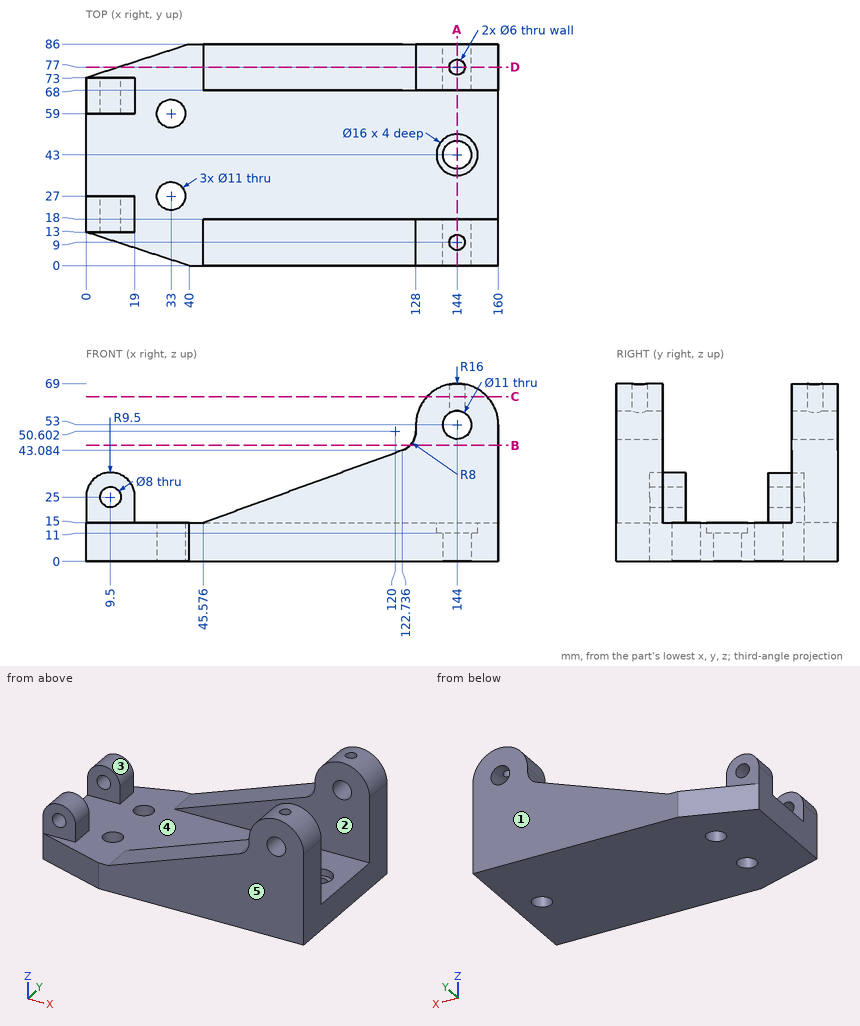
Part print with two shaded views. Sizes in mm from the minimum x, y, z corner. A direction names the side the tool comes from. Coordinates: 2 decimals unless noted, no trailing zeros. Loops run counter-clockwise (first coordinate to the right, second up) from the corner with the lowest first, then second, coordinate; pieces in that order, holes last. Notation, with made-up numbers: (-31.75, 77) -> (-22.75, 77) arc R13 cw to (-22.75, 81) -> close; hole circle Ø3 at (84.5, 21.25). An arc over 180 degrees is marked (long way). Answer as a JSON object with one key per item and string values.
Q1. Cut at B-B (z = 45). List the corners of the cut face in (x, y), and give its area (3 significant figures).
Report:
{"outline": "(125.71, 0) -> (160, 0) -> (160, 18) -> (125.71, 18) -> close; (125.71, 68) -> (160, 68) -> (160, 86) -> (125.71, 86) -> close", "area": "1,230 mm2"}
Q2. Cut at D-D (y = 77). List the corners of the cut face in (x, z) (1 decimal).
Report:
{"outline": "(12.3, 0) -> (160, 0) -> (160, 53) arc R16 ccw to (147, 68.7) -> (147, 57.6) arc R5.5 cw (long way) to (141, 57.6) -> (141, 68.7) arc R16 ccw to (128, 53) -> (128, 50.6) arc R8 cw to (122.7, 43.1) -> (45.6, 15) -> (12.3, 15) -> close"}
Q3. Pull direction Y, two halves, no side cores. Call the marked faces 3, 4 and 5: released by +Y, released by -Y, zero draft, split by the parting line, or undercut.
Report:
{"face 3": "zero draft", "face 4": "undercut", "face 5": "released by -Y"}
Q4. Cut at C-C (z = 64). List the corners of the cut face in (x, y).
Report:
{"outline": "(132.38, 0) -> (155.62, 0) -> (155.62, 18) -> (132.38, 18) -> close; (132.38, 68) -> (155.62, 68) -> (155.62, 86) -> (132.38, 86) -> close; hole circle Ø6 at (144, 9); hole circle Ø6 at (144, 77)"}
Q5. Probe probe 1 along Z at (x, y) = (9.5, 18.5); probe 2 along Y at (x, z) = (144, 64.25); probe 3 along Y at (x, z) = (108, 21). List the from-to ranges inside material, lowest first.
Report:
{"probe 1": "z = 0 to 21, 29 to 34.5", "probe 2": "y = 0 to 6, 12 to 18, 68 to 74, 80 to 86", "probe 3": "y = 0 to 18, 68 to 86"}
Q6. Cut at A-A (x = 144). State how many separate pieces and enclosed holes the cut face has, and give its area (3 significant figures).
Report:
{"separate pieces": "6", "enclosed holes": "0", "area": "2,530 mm2"}
Q7. Flat gauge pins, fed straight in: P1, Ø0.7, axis at y = 76.5, z = 52, coming from the -X side; P2, Ø9.5, axis at x = 11.5, z = 20.5, coming from the +Y side; P3, Ø14.5, axis at x = 33, y = 27, coming from the +Z side; P4, Ø9, axis at x = 144, z = 53, coming from the -Y side. Where does each tip first touch, or does it go through?
Report:
{"P1": "stops at x = 128", "P2": "stops at y = 73", "P3": "stops at z = 15", "P4": "passes through"}
Q8. 3-axis set-ups, long thin cutter, end or side, ignore diameter. For the marked faces 1 and 2: which of +Z, -Z, +X, -X, +Y, -Y reach the whole face in a straight line?
Report:
{"face 1": "+Z, -Z, +X, -X, +Y", "face 2": "+Z, +X"}
